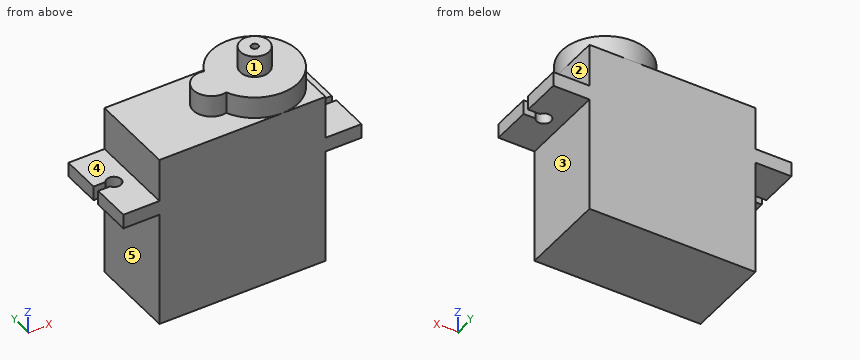
from build123d import *

# Parameters (mm, degrees)
F0_W      = 23
F0_H      = 12
F1_DEPTH  = 16
F2_W      = 33
F2_H      = 12
F3_DEPTH  = 2
F4_W      = 23
F4_H      = 12
F5_DEPTH  = 6
F7_DEPTH  = 3
F8_R      = 2
F9_DEPTH  = 3
F11_DEPTH = 18.001
F12_R     = 0.5
F13_DEPTH = 3


with BuildPart() as f1:
    # F0 (on Top) → F1 (new body)
    with BuildSketch(Plane.XY):
        Rectangle(F0_W, F0_H)
    extrude(amount=F1_DEPTH)

    # F2 (on face) → F3 (join)
    with BuildSketch(Plane.XY.offset(16)):
        Rectangle(F2_W, F2_H)
    extrude(amount=F3_DEPTH)

    # F4 (on face) → F5 (join)
    with BuildSketch(Plane.XY.offset(18)):
        Rectangle(F4_W, F4_H)
    extrude(amount=F5_DEPTH)

    # F6 (on face) → F7 (join)
    with BuildSketch(Plane.XY.offset(24)):
        with BuildLine():
            ThreePointArc((0.0208333333, -2.4451447071), (6.75, -5.8683472972), (11.5, 0))
            ThreePointArc((11.5, 0), (6.75, 5.8683472972), (0.0208333333, 2.4451447071))
            ThreePointArc((0.0208333333, 2.4451447071), (1.4432039694, 1.572882174), (2, 0))
            ThreePointArc((2, 0), (1.4432039694, -1.572882174), (0.0208333333, -2.4451447071))
        make_face()
        with BuildLine():
            ThreePointArc((2, 0), (1.4432039694, 1.572882174), (0.0208333333, 2.4451447071))
            ThreePointArc((0.0208333333, 2.4451447071), (-0.5, 0), (0.0208333333, -2.4451447071))
            ThreePointArc((0.0208333333, -2.4451447071), (1.4432039694, -1.572882174), (2, 0))
        make_face()
        with BuildLine():
            ThreePointArc((0.0208333333, -2.4451447071), (-0.5, 0), (0.0208333333, 2.4451447071))
            ThreePointArc((0.0208333333, 2.4451447071), (-3, 0), (0.0208333333, -2.4451447071))
        make_face()
    extrude(amount=F7_DEPTH)

    # F8 (on face) → F9 (join)
    with BuildSketch(Plane.XY.offset(27)):
        with Locations((5.5, 0)):
            Circle(F8_R)
    extrude(amount=F9_DEPTH)

    # F10 (on face) → F11 (cut, through all)
    with BuildSketch(Plane.XY.offset(18)):
        with BuildLine():
            ThreePointArc((-14.8660254038, -0.5), (-13.7411809549, -0.9659258263), (-13, 0))
            ThreePointArc((-13, 0), (-13.7411809549, 0.9659258263), (-14.8660254038, 0.5))
            Line((-14.8660254038, 0.5), (-14.8660254038, -0.5))
        make_face()
        with BuildLine():
            Line((-14.8660254038, -0.5), (-14.8660254038, 0.5))
            ThreePointArc((-14.8660254038, 0.5), (-15, 0), (-14.8660254038, -0.5))
        make_face()
        with BuildLine():
            ThreePointArc((-14.8660254038, -0.5), (-15, 0), (-14.8660254038, 0.5))
            Line((-14.8660254038, 0.5), (-16.5, 0.5))
            Line((-16.5, 0.5), (-16.5, -0.5))
            Line((-16.5, -0.5), (-14.8660254038, -0.5))
        make_face()
        with BuildLine():
            ThreePointArc((14.8660254038, -0.5), (14.9659258263, -0.2588190451), (15, 0))
            ThreePointArc((15, 0), (14.9659258263, 0.2588190451), (14.8660254038, 0.5))
            Line((14.8660254038, 0.5), (14.8660254038, -0.5))
        make_face()
        with BuildLine():
            ThreePointArc((14.8660254038, 0.5), (14.9659258263, 0.2588190451), (15, 0))
            ThreePointArc((15, 0), (14.9659258263, -0.2588190451), (14.8660254038, -0.5))
            Line((14.8660254038, -0.5), (16.5, -0.5))
            Line((16.5, -0.5), (16.5, 0.5))
            Line((16.5, 0.5), (14.8660254038, 0.5))
        make_face()
        with BuildLine():
            Line((14.8660254038, -0.5), (14.8660254038, 0.5))
            ThreePointArc((14.8660254038, 0.5), (13, 0), (14.8660254038, -0.5))
        make_face()
    extrude(amount=-F11_DEPTH, mode=Mode.SUBTRACT)

    # F12 (on face) → F13 (cut)
    with BuildSketch(Plane.XY.offset(30)):
        with Locations((5.5, 0)):
            Circle(F12_R)
    extrude(amount=-F13_DEPTH, mode=Mode.SUBTRACT)


solid = f1.part
Geometry: final body of the model. Coordinates: model frame, mm. Face numbers are marked on the shaded views. A direction names the side the tool comes from. Give positions to 0.01 mm unless a question says otherwise; leave off trailing zeros. Write each loop counter-clockwise with the first axis right and the second up, starting at its lowest first coordinate (ties: lowest second). Pieces come first, ordered by that corner, then holes. Notation, with made-up numbers: M 65,-28 L 77,-28 A22 ccw 77,5 Z; hole C 71,25 d10. An arc over 180 degrees is marked long. Answer in a Markdown table with one row per item. Add a question column.
(1) First-contact query: pin 1 (6.5 mm diameter, centred on y = 0.5, z = 21.5, fed in from -X); pin 2 (6 mm diameter, centred on y = -2, z = 7, fed in from +X); pin 3 (1.5 mm diameter, centred on x = -15, y = 1.5, fed in from +Z). Flat tips, straight axial feed; report the tip coordinate or a pass-through.
(2) Reachability of the marked faces 1, 2, 3, 4 and 5 from +Z, -Z, +X, -X, +Y, -Y: full face, straight path, thin tool, end or side. Return the list, or none.
(3) Section C-C on z = 18.5. Return loops of the section in (x, y).
(4) Section D-D on x = 7. Return loops of the section in (y, z), and give its area (3 significant figures).
(5) Section B-B on x = -0.5. Return loops of the section in (y, z), and give its area (3 significant figures).
(6) Ray query, line 1 (Y direction, x = 5.5, z = 29.45); line 2 (X direction, y = 5.75, z = 22.5); line 3 (Z direction, x = -10, y = -3.25). Return the intervals inside material, ascending.
(7) Section A-A on x = 14. Return loops of the section in (y, z).
Result set:
| question | item | result |
|---|---|---|
| 1 | pin 1 | stops at x = -11.5 |
| 1 | pin 2 | stops at x = 11.5 |
| 1 | pin 3 | stops at z = 18 |
| 2 | face 1 | +Z |
| 2 | face 2 | +Z, +X, +Y, -Y |
| 2 | face 3 | -Z, +X, +Y, -Y |
| 2 | face 4 | +Z, -X, +Y, -Y |
| 2 | face 5 | -Z, -X, +Y, -Y |
| 3 | outline | M -11.5,-6 L 11.5,-6 L 11.5,6 L -11.5,6 Z |
| 4 | outline | M -6,0 L 6,0 L 6,24 L 5.81,24 L 5.81,27 L 1.32,27 L 1.32,30 L -1.32,30 L -1.32,27 L -5.81,27 L -5.81,24 L -6,24 Z |
| 4 | area | 331 mm^2 |
| 5 | outline | M -6,0 L 6,0 L 6,24 L 2.5,24 L 2.5,27 L -2.5,27 L -2.5,24 L -6,24 Z |
| 5 | area | 303 mm^2 |
| 6 | line 1 | y = -2 to -0.5, 0.5 to 2 |
| 6 | line 2 | x = -11.5 to 11.5 |
| 6 | line 3 | z = 0 to 24 |
| 7 | outline | M -6,16 L -1,16 L -1,18 L -6,18 Z; M 1,16 L 6,16 L 6,18 L 1,18 Z |
